Design review of the part built by this model. Coordinates are the model's own, in mm. Face numbers are marked on the shaded views. A direction names the side the tool comes from. Give positions to 0.01 mm unless a question says otherwise; leave off trailing zeros. Loops run counter-clockwise (first coordinate to the right, second up) from the corner with the lowest first, then second, coordinate; pieces in that order, holes last.
from build123d import *

# Parameters (mm, degrees)
SKETCH_4_R          = 2.25
CUT_EXTRUDE_1_DEPTH = 65
SKETCH_5_R          = 3.75
CUT_EXTRUDE_4_DEPTH = 4.1
CUT_EXTRUDE_3_DEPTH = 65


with BuildPart() as part:
    # Sketch 1 → Revolve 1 (revolve)
    with BuildSketch(Plane.XY):
        Polygon((12, 24), (6, 24), (6, 14), (0, 14), (0, 10), (1.2, 10), (1.2, 8), (68.8, 8), (68.8, 10), (70, 10), (70, 14), (12, 14), align=None)
    revolve(axis=Axis((70, 0, 0), (-1, 0, 0)))

    # Sketch 4 → Cut-Extrude 1 (cut, through all)
    with BuildSketch(Plane.ZY.offset(-6)):
        with Locations((15.5, 11)):
            Circle(SKETCH_4_R)
        with Locations((-15.5, -11)):
            Circle(SKETCH_4_R)
        with Locations((-15.5, 11)):
            Circle(SKETCH_4_R)
        with Locations((15.5, -11)):
            Circle(SKETCH_4_R)
    extrude(amount=-CUT_EXTRUDE_1_DEPTH, mode=Mode.SUBTRACT)

    # Sketch 5 → Cut-Extrude 4 (cut)
    with BuildSketch(Plane.ZY.offset(-6)):
        with Locations((15.5, 11)):
            Circle(SKETCH_5_R)
        with Locations((-15.5, 11)):
            Circle(SKETCH_5_R)
        with Locations((-15.5, -11)):
            Circle(SKETCH_5_R)
        with Locations((15.5, -11)):
            Circle(SKETCH_5_R)
    extrude(amount=-CUT_EXTRUDE_4_DEPTH, mode=Mode.SUBTRACT)

    # Sketch 7 → Cut-Extrude 3 (cut, through all)
    with BuildSketch(Plane.ZY.offset(-6)):
        with BuildLine():
            Line((-16.941074346, 17), (16.941074346, 17))
            ThreePointArc((16.941074346, 17), (0, 24), (-16.941074346, 17))
        make_face()
        with BuildLine():
            Line((-16.941074346, -17), (16.941074346, -17))
            ThreePointArc((16.941074346, -17), (0, -24), (-16.941074346, -17))
        make_face()
    extrude(amount=-CUT_EXTRUDE_3_DEPTH, mode=Mode.SUBTRACT)


solid = part.part
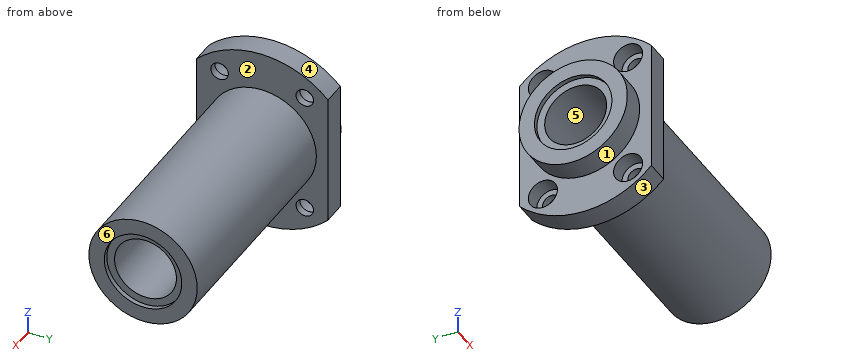
Q1. Insertion check: pin 1 (8 mm diameter, centred on y = 11, z = 16.5, fed in from -X); pin 2 (6 mm diameter, centred on y = -11, z = 15.5, fed in from -X); pin 3 (8 mm diameter, centred on x = 38.5, z = 5.5, fed in from +Y). Each pin has a flat end and moves straight along its axis. Give the tip position at first contact, or say it passes through.
Results:
pin 1: stops at x = 6
pin 2: stops at x = 10.1
pin 3: stops at y = 13.92
Q2. Draft analysis for pull direction Z (two halves, no side actions). For the marked faces 4, 5 and 6, state which applies: pulls with the +Z half, pulls with the -Z half, needs draft (parallel to the pull), parting line crosses it, or undercut.
Results:
face 4: pulls with the +Z half
face 5: undercut
face 6: needs draft
Q3. Wall thickness on line 1 (Z direction, x = 69.75, y = 0); line 2 (Y direction, x = 3, z = -0.5); line 3 (Z direction, x = 10, y = -9): over which ranges is each line inside the solid? List them lowest first.
Results:
line 1: z = -14 to -10, 10 to 14
line 2: y = -13.99 to -7.98, 7.98 to 13.99
line 3: z = -22.25 to -18.67, -12.33 to 12.33, 18.67 to 22.25
Q4. Take a section at C-C (z = 0). Give the boundary of the cut face in (x, y), plus the area to 3 significant figures.
Results:
outline: (0, -14) - (6, -14) - (6, -17) - (12, -17) - (12, -14) - (70, -14) - (70, -10) - (68.8, -10) - (68.8, -8) - (1.2, -8) - (1.2, -10) - (0, -10) - close; (0, 10) - (1.2, 10) - (1.2, 8) - (68.8, 8) - (68.8, 10) - (70, 10) - (70, 14) - (12, 14) - (12, 17) - (6, 17) - (6, 14) - (0, 14) - close
area: 866 mm2
Q5. Take a section at D-D (y = -11). Give the boundary of the cut face in (x, z), plus the area to 3 significant figures.
Results:
outline: (0, -8.66) - (6, -8.66) - (6, -11.75) - (10.1, -11.75) - (10.1, -13.25) - (12, -13.25) - (12, -8.66) - (70, -8.66) - (70, 8.66) - (12, 8.66) - (12, 13.25) - (10.1, 13.25) - (10.1, 11.75) - (6, 11.75) - (6, 8.66) - (0, 8.66) - close; (6, -21.33) - (12, -21.33) - (12, -17.75) - (10.1, -17.75) - (10.1, -19.25) - (6, -19.25) - close; (6, 19.25) - (10.1, 19.25) - (10.1, 17.75) - (12, 17.75) - (12, 21.33) - (6, 21.33) - close
area: 1,290 mm2
Q6. Take a section at B-B (y = -5.5). Give the boundary of the cut face in (x, z).
Results:
outline: (0, -12.87) - (6, -12.87) - (6, -23.36) - (12, -23.36) - (12, -12.87) - (70, -12.87) - (70, -8.35) - (68.8, -8.35) - (68.8, -5.81) - (1.2, -5.81) - (1.2, -8.35) - (0, -8.35) - close; (0, 8.35) - (1.2, 8.35) - (1.2, 5.81) - (68.8, 5.81) - (68.8, 8.35) - (70, 8.35) - (70, 12.87) - (12, 12.87) - (12, 23.36) - (6, 23.36) - (6, 12.87) - (0, 12.87) - close
Q7. Take a section at A-A (z = 15.5). Give the boundary of the cut face in (x, y), plus the area to 3 significant figures.
Results:
outline: (6, -17) - (12, -17) - (12, -13.25) - (10.1, -13.25) - (10.1, -14.75) - (6, -14.75) - close; (6, -7.25) - (10.1, -7.25) - (10.1, -8.75) - (12, -8.75) - (12, 8.75) - (10.1, 8.75) - (10.1, 7.25) - (6, 7.25) - close; (6, 14.75) - (10.1, 14.75) - (10.1, 13.25) - (12, 13.25) - (12, 17) - (6, 17) - close
area: 125 mm2
Q8. Tool access review of the marked faces 1, 2 and 3: name each direction out of +Z, -Z, +X, -X, +Y, -Y from which nothing blocks a thin tool from reaching the whole face with its end or side.
Results:
face 1: -X
face 2: +X
face 3: -Z, +X, -X
